Design review of the part built by this model. Coordinates are the model's own, in mm. Coordinates: 2 decimals unless noted, no trailing zeros. Loops run counter-clockwise (first coordinate to the right, second up) from the corner with the lowest first, then second, coordinate; pieces in that order, holes last.
Q1. Add section D-D on x = 20.5. Give the boundary of the cut face in (y, z).
Q2. For P1, Ø2.5, axis at x = 72.3, y = -21.52, coming from the +Z side; P2, Ø1, axis at y = 8, z = 1.5, coming from the +X side; P3, Ø1.5, axis at x = 114, z = 2, coming from the +Y side; P4, Ø0.9, axis at y = -9.5, z = 1, coming from the +X side, all flat-tipped, find the tip position at first contact; note any pin that passes through.
Q3. Wall thickness on probe 1 along Y at (x, z) = (73, 1.65); probe 2 along Y at (x, z) = (18.5, 1.95); probe 3 along Y at (x, z) = (9, 2.1): over which ranges is each line inside the solid? List them lowest first.
Q4. Add section A-A on x = 53. Give the boundary of the cut face in (y, z).
Q5. Add section B-B on z = 1.5. Give the boundary of the cut face in (x, y), and give its area (3 significant figures).
Q6. Add section C-C on y = 22.5. Give the boundary of the cut face in (x, z).
```python
from build123d import *

# Parameters (mm, degrees)
RESSALTO_EXTRUS_O1_DEPTH = 3
ESBO_O2_W                = 40.000247185
ESBO_O2_H                = 3
CORTE_EXTRUS_O1_DEPTH    = 147.710752088
ESBO_O3_R                = 1.5
CORTE_EXTRUS_O2_DEPTH    = 147.710752088


with BuildPart() as part:
    # Esboço1 → Ressalto-extrusão1 (new body)
    with BuildSketch(Plane.XY):
        with BuildLine():
            Line((-23.696540285, -59.026029985), (126.303641818, -59.026029985))
            Line((126.303641818, -59.026029985), (134.27116449, -59.022933245))
            Line((134.27116449, -59.022933245), (134.27116449, -19.822933247))
            ThreePointArc((134.27116449, -19.822933247), (131.52375333, -12.35888539), (124.30352468, -9.022933247))
            Line((124.30352468, -9.022933247), (108.30352468, -9.022933247))
            ThreePointArc((108.30352468, -9.022933247), (100.95374961, -5.803848113), (98.335884873, 1.780905469))
            ThreePointArc((98.335884873, 1.780905469), (60.482361862, 56.216031378), (-0.245391502, 29.603776524))
            ThreePointArc((-0.245391502, 29.603776524), (-0.409038284, 20.889653739), (6.32530272, 15.356899684))
            ThreePointArc((6.32530272, 15.356899684), (12.045479144, 14.777616646), (17.711135048, 15.755538086))
            ThreePointArc((17.711135048, 15.755538086), (22.936163149, 14.335796242), (23.805019321, 8.991483891))
            ThreePointArc((23.805019321, 8.991483891), (12.741533396, -4.118425729), (-3.696722505, -9.022933247))
            ThreePointArc((-3.696722505, -9.022933247), (-24.90992594, -17.809729811), (-33.696722505, -39.022933247))
            Line((-33.696722505, -39.022933247), (-33.696540284, -49.026212146))
            ThreePointArc((-33.696540284, -49.026212146), (-30.767543693, -56.0971622), (-23.696540285, -59.026029985))
        make_face()
    extrude(amount=RESSALTO_EXTRUS_O1_DEPTH)

    # Esboço2 → Corte-extrusão1 (cut, through all)
    with BuildSketch(Plane.XY.offset(3)):
        with Locations((60.303401088, -9.022933247)):
            Rectangle(ESBO_O2_W, ESBO_O2_H)
    extrude(amount=-CORTE_EXTRUS_O1_DEPTH, mode=Mode.SUBTRACT)

    # Esboço3 → Corte-extrusão2 (cut, through all)
    with BuildSketch(Plane.XY.offset(3)):
        with Locations((72.30352468, 3.477066753)):
            Circle(ESBO_O3_R)
        with Locations((72.30352468, -21.522933247)):
            Circle(ESBO_O3_R)
    extrude(amount=-CORTE_EXTRUS_O2_DEPTH, mode=Mode.SUBTRACT)


solid = part.part
```
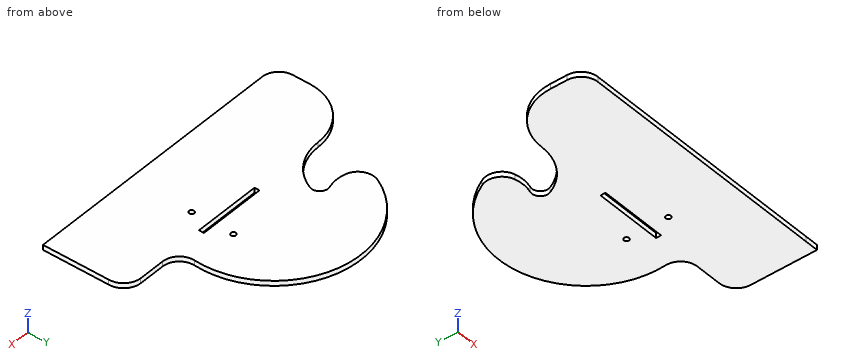
Entries:
1. outline: (-59.03, 0) - (3.24, 0) - (3.24, 3) - (-59.03, 3) - close; (15.82, 0) - (51.36, 0) - (51.36, 3) - (15.82, 3) - close
2. P1: passes through
2. P2: stops at x = 98.48
2. P3: stops at y = -9.02
2. P4: stops at x = 128.2
3. probe 1: y = -59.03 to -22.85, -20.19 to -10.52, -7.52 to 2.15, 4.81 to 50.84
3. probe 2: y = -59.03 to 0.8, 15.94 to 50.16
3. probe 3: y = -59.03 to -6.2, 14.89 to 42.49
4. outline: (-59.03, 0) - (-10.52, 0) - (-10.52, 3) - (-59.03, 3) - close; (-7.52, 0) - (57.75, 0) - (57.75, 3) - (-7.52, 3) - close
5. outline: (-33.7, -49.03) arc R10 ccw to (-23.7, -59.03) - (126.3, -59.03) - (134.27, -59.02) - (134.27, -19.82) arc R10.39 ccw to (124.3, -9.02) - (108.3, -9.02) arc R10 cw to (98.34, 1.78) arc R52.2 ccw to (-0.25, 29.6) arc R10 ccw to (6.33, 15.36) arc R21.21 ccw to (17.71, 15.76) arc R5 cw to (23.81, 8.99) arc R30 cw to (-3.7, -9.02) arc R30 ccw to (-33.7, -39.02) - close; hole (40.3, -10.52) - (80.3, -10.52) - (80.3, -7.52) - (40.3, -7.52) - close; hole circle Ø3 at (72.3, -21.52); hole circle Ø3 at (72.3, 3.48)
5. area: 13,300 mm2
6. outline: (-0.99, 0) - (95.82, 0) - (95.82, 3) - (-0.99, 3) - close
